Input: part model. Units: mm. Frame: model coordinates. A direction names the side the tool comes from. Coordinates: 2 decimals unless noted, no trailing zeros. Loops run counter-clockwise (first coordinate to the right, second up) from the corner with the lowest first, then second, coordinate; pieces in that order, holes last.
```python
from build123d import *

# Parameters (mm, degrees)
SKETCH1_W           = 95.25
SKETCH1_H           = 3.175
BOSS_EXTRUDE1_DEPTH = 12.7
SKETCH2_R           = 1.89865
CUT_EXTRUDE1_DEPTH  = 12.7
SKETCH3_W           = 92.857106726
SKETCH3_H           = 7.363806504
BOSS_EXTRUDE2_DEPTH = 0.000254


with BuildPart() as part:
    # Sketch1 → Boss-Extrude1 (new body)
    with BuildSketch(Plane.XY):
        Rectangle(SKETCH1_W, SKETCH1_H)
        Polygon((47.625, 1.5875), (47.625, -1.5875), (50.8, -1.5875), (50.8, 11.1125), (47.625, 11.1125), align=None)
    extrude(amount=BOSS_EXTRUDE1_DEPTH)

    # Sketch2 → Cut-Extrude1 (cut)
    with BuildSketch(Plane.ZY.offset(-47.625)):
        with Locations((3.175, 6.35)):
            Circle(SKETCH2_R)
        with Locations((9.525, 6.35)):
            Circle(SKETCH2_R)
    extrude(amount=-CUT_EXTRUDE1_DEPTH, mode=Mode.SUBTRACT)

    # Sketch3 → Boss-Extrude2 (add)
    with BuildSketch(Plane(origin=(0, 1.5875, 0), x_dir=(1, 0, 0), z_dir=(0, 1, 0))):
        with Locations((0, -6.35)):
            Rectangle(SKETCH3_W, SKETCH3_H)
    extrude(amount=BOSS_EXTRUDE2_DEPTH)


solid = part.part
```
Item 1: Section query A-A (y = 6.35). Output: boundary loops of the cut face in (x, z) (3 decimals), then the cut area to 3 significant figures.
Result:
outline: (47.625, 0) - (50.8, 0) - (50.8, 1.276) - (47.625, 1.276) - close; (47.625, 5.074) - (50.8, 5.074) - (50.8, 7.626) - (47.625, 7.626) - close; (47.625, 11.424) - (50.8, 11.424) - (50.8, 12.7) - (47.625, 12.7) - close
area: 16.2 mm2
Item 2: Mould query, pull axis Y, two halves, no side actions, for faces 1 (the face through (-1, 1.588, 6)), 2 (the face through (49.19, 6.43, 7.63)), 3 (the face through (49.19, 4.666, 4.051)), 4 (the face through (5, 1, 12.7)). Classes: +Y half, -Y half, draft (parallel to the pull), parting line (faces both ways), or undercut.
Result:
face 1: +Y half
face 2: undercut
face 3: undercut
face 4: draft
Item 3: Line query: L1, parallel to Y at x = -41, z = 8.75; L2, parallel to X at y = 9.75, z = 3 (3 decimals). Output: solid intervals per line, ascending.
Result:
L1: y = -1.59 to 1.59
L2: x = 47.625 to 50.8
Item 4: Contact query for flat-ended pins moving along their axis: P1, Ø6.5, axis at x = -14.5, z = 5, coming from the +Y side; P2, Ø3, axis at y = 4.5, z = 6.5, coming from the -X side (3 decimals); P3, Ø3.5, axis at y = 6.35, z = 3.175, coming from the +X side (3 decimals). Output: stop coordinate, or through.
Result:
P1: stops at y = 1.59
P2: stops at x = 47.625
P3: passes through
Item 5: Reachability of faces 5 (the face through (-47.625, 0, 6)), 6 (the face through (-1, 1.588, 2)) from +Z, -Z, +X, -X, +Y, -Y: full face, straight path, thin tool, end or side. Return the list, or none.
Result:
face 5: +Z, -Z, -X, +Y, -Y
face 6: +Z, -Z, -X, +Y
